Job drawing, mm, ordinate dimensions from the low corner. One solid piece. A direction names the side the tool comes from. Give positions to 0.01 mm unless a question says otherwise; leave off trailing zeros. Loops run counter-clockwise (first coordinate to the right, second up) from the corner with the lowest first, then second, coordinate; pieces in that order, holes last. Notation, with made-up numbers: (82, 15) -> (126, 15) arc R26 ccw to (126, 51) -> close; hole circle Ø7 at (33.5, 41). An arc over 180 degrees is marked (long way). Answer as a JSON object with one key per item and string values. Group by question number.
Q1. Band-saw the part on B-B, the plane x = 40. Write the cut outline in (y, z), plus the area to 3 significant figures.
Q2. Band-saw the part on D-D, the plane y = 23.5. Write the cut outline in (x, z).
Q3. Tool access for the marked faces 1, 2, 3 and 4: list every direction of +Z, -Z, +X, -X, +Y, -Y with a clear straight run to the whole face (end or side of a thin tool).
Q4. Wall check: probe 1 along X at (y, z) = (17, 18.6); probe 2 along Y at (x, z) = (3.5, 18.3); probe 3 along X at (y, z) = (4, 6.25). Give the ranges that are in metal, low to high. Write a range as from..to.
Q5. Drop flat-ended pins along their axis: pin 1 (3 mm diameter, centred on x = 41.5, y = 17, fed in from -Z); pin 2 (1.5 mm diameter, centred on y = 24.5, z = 3.5, fed in from -X); pin 3 (3.5 mm diameter, centred on x = 42, y = 17.5, fed in from -Z); pin 4 (1.1 mm diameter, centred on x = 39, z = 18.5, fed in from +Y). Give the stop position or say it passes through.
Q6. Band-saw the part on A-A, the plane z = 18.5. Write the cut outline in (x, y), plus the area to 3 significant figures.
Q7. Band-saw the part on C-C, the plane z = 10.5. Write the cut outline in (x, y).
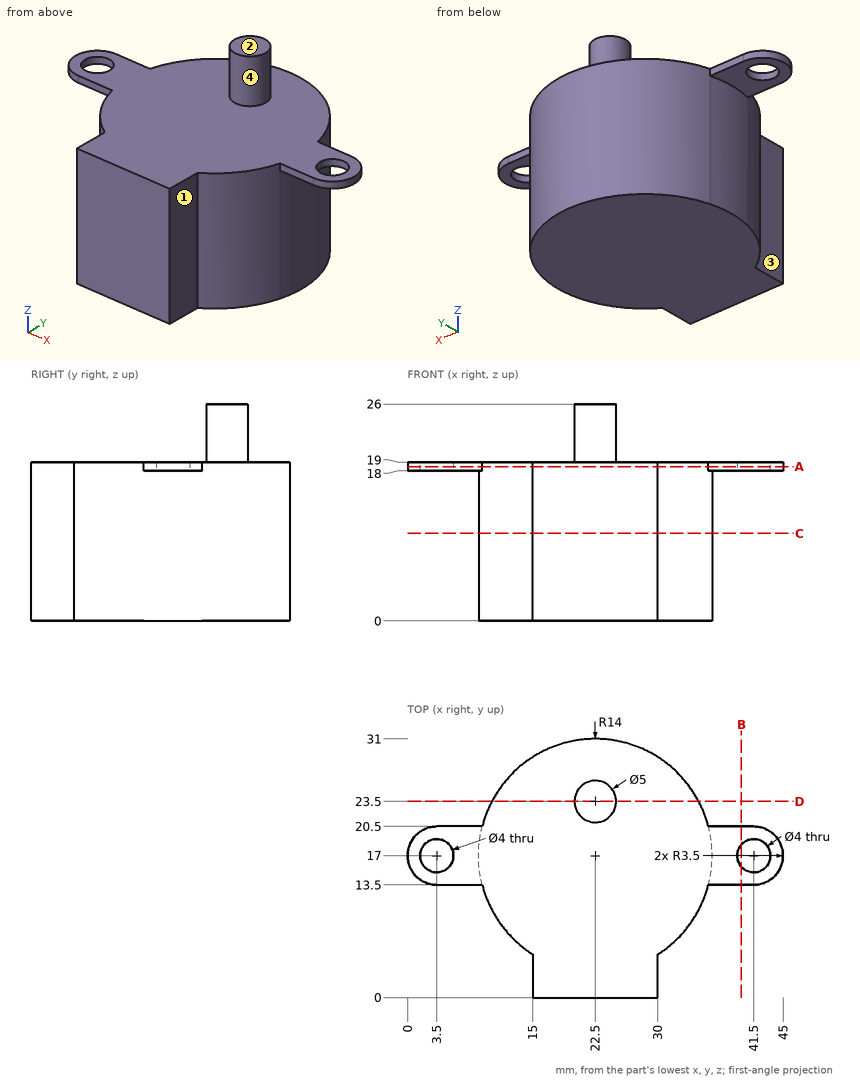
Worked answers:
{
 "1": {"outline": "(13.5, 18) -> (15.68, 18) -> (15.68, 19) -> (13.5, 19) -> close; (18.32, 18) -> (20.5, 18) -> (20.5, 19) -> (18.32, 19) -> close", "area": "4.35 mm2"},
 "2": {"outline": "(10.1, 0) -> (34.9, 0) -> (34.9, 19) -> (25, 19) -> (25, 26) -> (20, 26) -> (20, 19) -> (10.1, 19) -> close"},
 "3": {"face 1": "+Z, -Z, +X, -Y", "face 2": "+Z, +X, -X, +Y, -Y", "face 3": "+Z, -Z, -X, -Y", "face 4": "+Z"},
 "4": {"probe 1": "0..1.5, 5.5..39.5, 43.5..45", "probe 2": "13.5..15, 19..20.5", "probe 3": "15..30"},
 "5": {"pin 1": "through", "pin 2": "x = 10.23", "pin 3": "z = 18", "pin 4": "y = 20.5"},
 "6": {"outline": "(3.5, 13.5) -> (8.94, 13.5) arc R14 ccw to (15, 5.18) -> (15, 0) -> (30, 0) -> (30, 5.18) arc R14 ccw to (36.06, 13.5) -> (41.5, 13.5) arc R3.5 ccw to (41.5, 20.5) -> (36.06, 20.5) arc R14 ccw to (8.94, 20.5) -> (3.5, 20.5) arc R3.5 ccw to start; hole circle Ø4 at (3.5, 17); hole circle Ø4 at (41.5, 17)", "area": "757 mm2"},
 "7": {"outline": "(15, 0) -> (30, 0) -> (30, 5.18) arc R14 ccw (long way) to (15, 5.18) -> close"}
}
